Verification items for this drawing (mm, ordinates from the low corner). Give positions to 0.01 mm unless a question says otherwise; leave off trailing zeros. Loops run counter-clockwise (first coordinate to the right, second up) from the corner with the lowest first, then second, coordinate; pieces in that order, holes last. Notation, with made-up numbers: (79, -11.75) - (108, -11.75) arc R17 cw to (108, 11.25) - close; hole circle Ø4 at (-4.75, 63.25). An arc over 180 degrees is marked (long way). Write item = value, one per line. Start each with the question number.
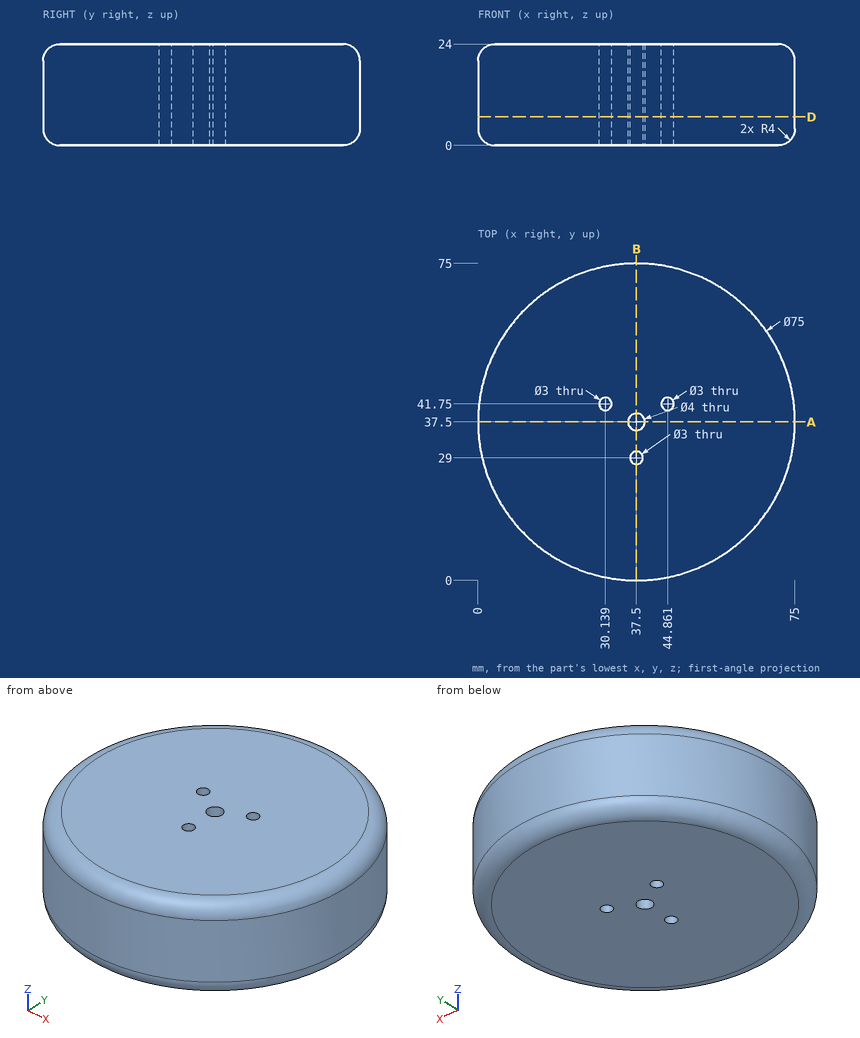
1) Cross-section at B-B on x = 37.5. Give the number of separate pieces and of enclosed holes in the cut face, and give its area (3 significant figures).
2) Gauge pin test, flat ends, axial feed: P1, Ø5, axis at y = 63, z = 3, coming from the +X side; P2, Ø10, axis at x = 48, z = 9, coming from the +Y side; P3, Ø8, axis at y = 10.5, z = 3.5, coming from the -X side; P4, Ø2.5, axis at x = 30.14, y = 41.75, coming from the +Z side. Record the tip position at first contact, or that the pin passes through.
3) Material ranges on line 1 along Y through (x, z) = (37.5, 5); line 2 along X through (y, z) = (41.75, 19.25); line 3 along Y through (x, z) = (14.5, 18), recorded low to high.
4) Cross-section at D-D on z = 6.75. Enter the section's corners in (x, y), and give its area (3 significant figures).
5) Cross-section at A-A on y = 37.5. Enter the section's corners in (x, z), and give its area (3 significant figures).
Checked values:
q1.separate_pieces = 3
q1.enclosed_holes = 0
q1.area = 1,620 mm²
q2.P1 = 67.04
q2.P2 = 74.59
q2.P3 = 7.9
q2.P4 = through
q3.line_1 = 0 to 27.5, 30.5 to 35.5, 39.5 to 75
q3.line_2 = 0.24 to 28.64, 31.64 to 43.36, 46.36 to 74.76
q3.line_3 = 7.88 to 67.12
q4.outline = circle Ø75 at (37.5, 37.5); hole circle Ø3 at (30.14, 41.75); hole circle Ø4 at (37.5, 37.5); hole circle Ø3 at (37.5, 29); hole circle Ø3 at (44.86, 41.75)
q4.area = 4,380 mm²
q5.outline = (0, 4) arc R4 ccw to (4, 0) - (35.5, 0) - (35.5, 24) - (4, 24) arc R4 ccw to (0, 20) - close; (39.5, 0) - (71, 0) arc R4 ccw to (75, 4) - (75, 20) arc R4 ccw to (71, 24) - (39.5, 24) - close
q5.area = 1,690 mm²
